Input: part model. Units: mm. Frame: model coordinates. Face numbers are marked on the shaded views. A direction names the side the tool comes from. Round coordinates to 2 decimals unless told otherwise and drop trailing zeros. Loops run counter-clockwise (first coordinate to the right, second up) from the corner with the lowest first, then second, coordinate; pieces in that order, holes last. Notation, with made-up numbers: (39, 77) -> (46, 77) arc R9 cw to (46, 81) -> close; hole circle Ø7 at (77, -4). An arc over 180 degrees is marked (long way). Answer as a JSON object with one key per item and string values. Group by question number.
Item 1: Section query D-D on x = -3.5. Return loops of the section in (y, z), and give its area (3 significant figures).
Item 2: Section query C-C on z = 4.25. Return loops of the section in (x, y).
Item 3: Material intervals for line 1 (Y direction, x = 0, z = 8); line 2 (Z direction, x = 6, y = 13.5); line 3 (Y direction, x = 7, z = 4.5), sorted ascending. Write a range as [from, to].
Item 4: Pin query (flat end, axial travel): pin 1 (4 mm diameter, centred on y = 10.5, z = 1.5, fed in from -X); pin 2 (2.5 mm diameter, centred on x = 7, y = 0, fed in from +Z); pin 3 (1.5 mm diameter, centred on y = -2, z = 5.5, fed in from +X); pin 4 (1.5 mm diameter, centred on x = 9.5, z = 8.5, fed in from -Y). Return the tip coordinate at first contact, or that it passes through.
Item 5: Draft query along X for the marked faces 4, 5 and 6. Return one class per face: released by +X, released by -X, zero draft, split by the parting line, or undercut.
Item 6: Section query B-B on x = 2. Return loops of the section in (y, z), and give its area (3 significant figures).
Item 7: Set-up query: the marked faces 1, 2 and 3. Return all of +Z, -Z, +X, -X, +Y, -Y with unobstructed straight access to the full face (end or side cutting, diameter ignored); none if empty.
Item 8: Section query A-A on y = 0. Return loops of the section in (x, z).
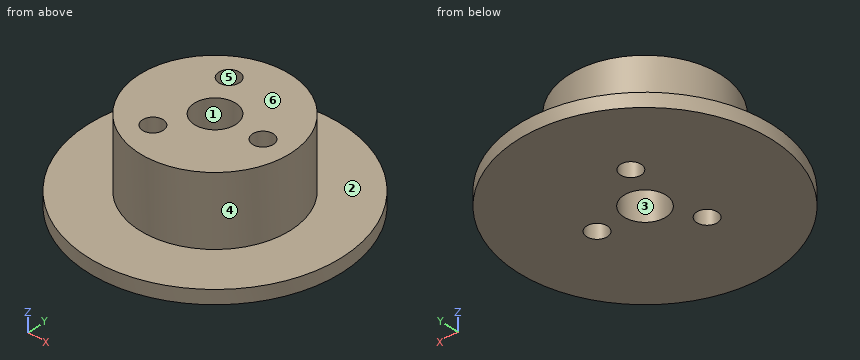
from build123d import *

# Parameters (mm, degrees)
SKETCH1_R           = 18.5
BOSS_EXTRUDE1_DEPTH = 3
SKETCH2_R           = 11
BOSS_EXTRUDE2_DEPTH = 2.5
SKETCH4_R           = 3.05
CUT_EXTRUDE1_DEPTH  = 27.734808771
SKETCH7_R           = 11
SKETCH7_R_2         = 3
BOSS_EXTRUDE3_DEPTH = 6.6
SKETCH9_R           = 1.5
CUT_EXTRUDE4_DEPTH  = 29.825509536
CUT_EXTRUDE5_START  = -1
SKETCH10_R          = 18.5
SKETCH10_R_2        = 11
CUT_EXTRUDE5_DEPTH  = 1


with BuildPart() as part:
    # Sketch1 → Boss-Extrude1 (new body)
    with BuildSketch(Plane.XY):
        Circle(SKETCH1_R)
    extrude(amount=BOSS_EXTRUDE1_DEPTH)

    # Sketch2 → Boss-Extrude2 (add)
    with BuildSketch(Plane.XY.offset(3)):
        Circle(SKETCH2_R)
    extrude(amount=BOSS_EXTRUDE2_DEPTH)

    # Sketch4 → Cut-Extrude1 (cut, through all)
    with BuildSketch(Plane(origin=(0, 0, 0), x_dir=(-1, 0, 0), z_dir=(0, 0, -1))):
        Circle(SKETCH4_R)
    extrude(amount=-CUT_EXTRUDE1_DEPTH, mode=Mode.SUBTRACT)

    # Sketch7 → Boss-Extrude3 (add)
    with BuildSketch(Plane.XY.offset(5.5)):
        Circle(SKETCH7_R)
        Circle(SKETCH7_R_2, mode=Mode.SUBTRACT)
    extrude(amount=BOSS_EXTRUDE3_DEPTH)

    # Sketch9 → Cut-Extrude4 (cut, through all)
    with BuildSketch(Plane.XY.offset(12.1)):
        with Locations((7, 0)):
            Circle(SKETCH9_R)
        with Locations((-3.5, -6.062177826)):
            Circle(SKETCH9_R)
        with Locations((-3.5, 6.062177826)):
            Circle(SKETCH9_R)
    extrude(amount=-CUT_EXTRUDE4_DEPTH, mode=Mode.SUBTRACT)

    # Sketch10 → Cut-Extrude5 (cut)
    with BuildSketch(Plane.XY.offset(3).offset(CUT_EXTRUDE5_START)):
        Circle(SKETCH10_R)
        Circle(SKETCH10_R_2, mode=Mode.SUBTRACT)
    extrude(amount=CUT_EXTRUDE5_DEPTH, mode=Mode.SUBTRACT)


solid = part.part
Solved:
{
 "1": {"outline": "(-18.17, 0) -> (-7.56, 0) -> (-7.56, 12.1) -> (-10.43, 12.1) -> (-10.43, 2) -> (-18.17, 2) -> close; (-4.56, 0) -> (4.56, 0) -> (4.56, 12.1) -> (-4.56, 12.1) -> close; (7.56, 0) -> (18.17, 0) -> (18.17, 2) -> (10.43, 2) -> (10.43, 12.1) -> (7.56, 12.1) -> close", "area": "211 mm²"},
 "2": {"outline": "circle Ø22 at (0, 0); hole circle Ø3 at (-3.5, -6.06); hole circle Ø3 at (-3.5, 6.06); hole circle Ø6.1 at (0, 0); hole circle Ø3 at (7, 0)"},
 "3": {"line 1": "[-11, -3], [3, 11]", "line 2": "[0, 2]", "line 3": "[-8.49, -1.5], [1.5, 8.49]"},
 "4": {"pin 1": "x = -16.43", "pin 2": "through", "pin 3": "x = 10.93", "pin 4": "y = -6.67"},
 "5": {"face 4": "split by the parting line", "face 5": "undercut", "face 6": "zero draft"},
 "6": {"outline": "(-18.39, 0) -> (-2.3, 0) -> (-2.3, 5.5) -> (-2.24, 5.5) -> (-2.24, 12.1) -> (-10.82, 12.1) -> (-10.82, 2) -> (-18.39, 2) -> close; (2.24, 5.5) -> (2.3, 5.5) -> (2.3, 0) -> (18.39, 0) -> (18.39, 2) -> (10.82, 2) -> (10.82, 12.1) -> (2.24, 12.1) -> close", "area": "237 mm²"},
 "7": {"face 1": "+Z, -Z", "face 2": "+Z", "face 3": "-Z"},
 "8": {"outline": "(-18.5, 0) -> (-3.05, 0) -> (-3.05, 5.5) -> (-3, 5.5) -> (-3, 12.1) -> (-11, 12.1) -> (-11, 2) -> (-18.5, 2) -> close; (3, 5.5) -> (3.05, 5.5) -> (3.05, 0) -> (5.5, 0) -> (5.5, 12.1) -> (3, 12.1) -> close; (8.5, 0) -> (18.5, 0) -> (18.5, 2) -> (11, 2) -> (11, 12.1) -> (8.5, 12.1) -> close"}
}
